Autodesk Inventor part; units mm, degrees
ref_plane "YZ Plane" through (0, 0, 0) normal (1, 0, 0) x (0, 1, 0)
ref_plane "XZ Plane" through (0, 0, 0) normal (0, 1, 0) x (-1, 0, 0)
ref_plane "XY Plane" through (0, 0, 0) normal (0, 0, 1) x (1, 0, 0)
sketch "Sketch1" plane through (0, 0, 0) normal (1, 0, 0) x (0, 1, 0)
  circle A0 centre (0, 0) radius 10.9
  circle A1 centre (0, 0) radius 1
  circle A2 centre (0, 0) radius 7
  circle A3 centre (7, 0) radius 1
  circle A4 centre (0, 7) radius 1
  circle A5 centre (-7, 0) radius 1
  circle A6 centre (0, -7) radius 1
  dimension "d2" = 14
  dimension "d0" = 21.8
  dimension "d1" = 2
  dimension "d3" = 2
  dimension "d6" = 360
extrude "Extrusion1" add sketch "Sketch1" along normal blind 2.8 contours A0 | A3 A2 A6 A5 A4
sketch "Sketch2" plane through (0, 0, 0) normal (-1, 0, 0) x (0, 0, 1)
  circle A0 centre (0, 0) radius 3.5
  line L0 (-0.0024, 0.0008) -> (1.8342, 0.0008) construction
  line L1 (0, 0) -> (2, 0) construction
  circle A1 centre (0, 0) radius 1.8335
  line L2 (-0.517, -1.932) -> (-0.6271, -1.7229)
  line L3 (-0.517, -1.932) -> (-0.3208, -1.8052)
  line L4 (-0.1736, -1.9924) -> (-0.3184, -1.8056)
  line L5 (-0.1736, -1.9924) -> (-0.0025, -1.8335)
  line L6 (0.175, -1.9923) -> (0, -1.8335)
  line L7 (0.175, -1.9923) -> (0.316, -1.806)
  line L8 (0.5183, -1.9317) -> (0.3184, -1.8056)
  line L9 (0.5183, -1.9317) -> (0.6248, -1.7237)
  line L10 (0.8458, -1.8123) -> (0.6271, -1.7229)
  line L11 (0.8458, -1.8123) -> (0.9146, -1.5891)
  line L12 (1.1477, -1.6379) -> (0.9167, -1.5878)
  line L13 (1.1477, -1.6379) -> (1.1766, -1.4061)
  line L14 (1.4147, -1.4137) -> (1.1785, -1.4045)
  line L15 (1.4147, -1.4137) -> (1.4029, -1.1804)
  line L16 (1.6387, -1.1466) -> (1.4045, -1.1785)
  line L17 (1.6387, -1.1466) -> (1.5866, -0.9189)
  line L18 (1.8129, -0.8446) -> (1.5878, -0.9167)
  line L19 (1.8129, -0.8446) -> (1.7221, -0.6294)
  line L20 (1.932, -0.517) -> (1.7229, -0.6271)
  line L21 (1.932, -0.517) -> (1.8052, -0.3208)
  line L22 (1.9924, -0.1736) -> (1.8056, -0.3184)
  line L23 (1.9924, -0.1736) -> (1.8335, -0.0025)
  line L24 (1.9923, 0.175) -> (1.8335, 0)
  line L25 (1.9923, 0.175) -> (1.806, 0.316)
  line L26 (1.9317, 0.5183) -> (1.8056, 0.3184)
  line L27 (1.9317, 0.5183) -> (1.7237, 0.6248)
  line L28 (1.8123, 0.8458) -> (1.7229, 0.6271)
  line L29 (1.8123, 0.8458) -> (1.5891, 0.9146)
  line L30 (1.6379, 1.1477) -> (1.5878, 0.9167)
  line L31 (1.6379, 1.1477) -> (1.4061, 1.1766)
  line L32 (1.4137, 1.4147) -> (1.4045, 1.1785)
  line L33 (1.4137, 1.4147) -> (1.1804, 1.4029)
  line L34 (1.1466, 1.6387) -> (1.1785, 1.4045)
  line L35 (1.1466, 1.6387) -> (0.9189, 1.5866)
  line L36 (0.8446, 1.8129) -> (0.9167, 1.5878)
  line L37 (0.8446, 1.8129) -> (0.6294, 1.7221)
  line L38 (0.517, 1.932) -> (0.6271, 1.7229)
  line L39 (0.517, 1.932) -> (0.3208, 1.8052)
  line L40 (0.1736, 1.9924) -> (0.3184, 1.8056)
  line L41 (0.1736, 1.9924) -> (0.0025, 1.8335)
  line L42 (-0.175, 1.9923) -> (0, 1.8335)
  line L43 (-0.175, 1.9923) -> (-0.316, 1.806)
  line L44 (-0.5183, 1.9317) -> (-0.3184, 1.8056)
  line L45 (-0.5183, 1.9317) -> (-0.6248, 1.7237)
  line L46 (-0.8458, 1.8123) -> (-0.6271, 1.7229)
  line L47 (-0.8458, 1.8123) -> (-0.9146, 1.5891)
  line L48 (-1.1477, 1.6379) -> (-0.9167, 1.5878)
  line L49 (-1.1477, 1.6379) -> (-1.1766, 1.4061)
  line L50 (-1.4147, 1.4137) -> (-1.1785, 1.4045)
  line L51 (-1.4147, 1.4137) -> (-1.4029, 1.1804)
  line L52 (-1.6387, 1.1466) -> (-1.4045, 1.1785)
  line L53 (-1.6387, 1.1466) -> (-1.5866, 0.9189)
  line L54 (-1.8129, 0.8446) -> (-1.5878, 0.9167)
  line L55 (-1.8129, 0.8446) -> (-1.7221, 0.6294)
  line L56 (-1.932, 0.517) -> (-1.7229, 0.6271)
  line L57 (-1.932, 0.517) -> (-1.8052, 0.3208)
  line L58 (-1.9924, 0.1736) -> (-1.8056, 0.3184)
  line L59 (-1.9924, 0.1736) -> (-1.8335, 0.0025)
  line L60 (-1.9923, -0.175) -> (-1.8335, 0)
  line L61 (-1.9923, -0.175) -> (-1.806, -0.316)
  line L62 (-1.9317, -0.5183) -> (-1.8056, -0.3184)
  line L63 (-1.9317, -0.5183) -> (-1.7237, -0.6248)
  line L64 (-1.8123, -0.8458) -> (-1.7229, -0.6271)
  line L65 (-1.8123, -0.8458) -> (-1.5891, -0.9146)
  line L66 (-1.6379, -1.1477) -> (-1.5878, -0.9167)
  line L67 (-1.6379, -1.1477) -> (-1.4061, -1.1766)
  line L68 (-1.4137, -1.4147) -> (-1.4045, -1.1785)
  line L69 (-1.4137, -1.4147) -> (-1.1804, -1.4029)
  line L70 (-1.1466, -1.6387) -> (-1.1785, -1.4045)
  line L71 (-1.1466, -1.6387) -> (-0.9189, -1.5866)
  line L72 (-0.8446, -1.8129) -> (-0.9167, -1.5878)
  line L73 (-0.8446, -1.8129) -> (-0.6294, -1.7221)
  arc A2 (2, 0) -> (1.9998, 0.0261) centre (0, 0) ccw
  point P0 (1.8335, 0)
  dimension "d10" = 7
  dimension "d13" = 360
extrude "Extrusion2" add sketch "Sketch2" along normal blind 2.2
thread "Thread1"
thread "Thread2"
thread "Thread3"
thread "Thread4"
thread "Thread5"
properties part number "Part R"
The model under review builds one solid part; all positions refer to its coordinate system, in mm. A direction names the side the tool comes from. Round coordinates to 2 decimals unless told otherwise and drop trailing zeros. Order: outer loops, then holes, each group sorted by start corner. A loop starts at its lowest first (then second) coordinate and runs counter-clockwise, first axis right, second up.
(1) Mouldability with a two-part tool opening along Z and no side actions: class faces 1 (the face through (-2.2, -2, 2)), 2 (the face through (1, 0, -8)), 3 (the face through (-1.085, 1.341, 3.233)) as released by +Z, released by -Z, zero draft, split by the parting line, or undercut.
Working result:
face 1: zero draft
face 2: undercut
face 3: split by the parting line
(2) Take a section at A-A, the plane x = 2.55. State the section outline as (y, z) points, plus the area to 3 significant figures.
Working result:
outline: circle Ø21.8 at (0, 0); hole circle Ø2 at (-7, 0); hole circle Ø2 at (0, -7); hole circle Ø2 at (0, 0); hole circle Ø2 at (0, 7); hole circle Ø2 at (7, 0)
area: 358 mm2
(3) Tool access review of faces 4 (the face through (0, 1, -1)), 5 (the face through (1.4, 6.2, 0.6)): name each direction out of +Z, -Z, +X, -X, +Y, -Y from which nothing blocks a thin tool from reaching the whole face with its end or side.
Working result:
face 4: -X
face 5: +X, -X
(4) Take a section at B-B, the plane y = 7. State the section outline as (x, z) points, plus the area to 3 significant figures.
Working result:
outline: (0, -8.36) - (2.8, -8.36) - (2.8, -1) - (0, -1) - close; (0, 1) - (2.8, 1) - (2.8, 8.36) - (0, 8.36) - close
area: 41.2 mm2
(5) For P1, Ø1.2, axis at y = -1, z = 0, coming from the -X side; P2, Ø2, axis at x = 1.5, z = -5, coming from the -Y side, all flat-tipped, find the tip position at first contact; note any pin that passes through.
Working result:
P1: stops at x = 0
P2: stops at y = -10.14
(6) Wall thickness on L1, parallel to Z at x = 1.6, y = 0; L2, parallel to X at y = 7.25, z = 7.75; L3, parallel to Z at x = 2.25, y = 7: over which ranges is each line inside the solid? List them lowest first.
Working result:
L1: z = -10.9 to -8, -6 to -1, 1 to 6, 8 to 10.9
L2: x = 0 to 2.8
L3: z = -8.36 to -1, 1 to 8.36
(7) Take a section at C-C, the plane z = -6.5. State the section outline as (x, y) points, plus the area to 3 significant figures.
Working result:
outline: (0, -8.75) - (2.8, -8.75) - (2.8, -0.87) - (0, -0.87) - close; (0, 0.87) - (2.8, 0.87) - (2.8, 8.75) - (0, 8.75) - close
area: 44.1 mm2
